Part model, mm, in its own coordinate system. Face numbers are marked on the shaded views. A direction names the side the tool comes from. Coordinates: 2 decimals unless noted, no trailing zeros. Order: outer loops, then holes, each group sorted by start corner. A loop starts at its lowest first (then second) coordinate and runs counter-clockwise, first axis right, second up. Notation, with made-up numbers: (14, 87.25) - (36, 87.25) arc R30 cw to (36, 110.25) - close; hole circle Ø5 at (7.5, -34). An arc over 180 degrees is marked (long way). Use a Markdown table: item, result. Add a question column.
1) Saw through at A-A on x = 44. List the corners of the cut face in (y, z), then the cut area to 3 significant figures.
2) Tool access for the marked faces 1, 2, 3, 4 and 5: list every direction of +Z, -Z, +X, -X, +Y, -Y with a clear straight run to the whole face (end or side of a thin tool).
3) Saw through at B-B on z = 10. List the corners of the cut face in (x, y).
4) Saw through at D-D on x = 30. List the corners of the cut face in (y, z), then the cut area to 3 significant figures.
5) Wall check: L1, parallel to X at y = 34.95, z = 15; L2, parallel to Z at x = 44, y = 34.15; L3, parallel to Y at x = 25.5, z = 16.5. Give the ranges that are in metal, low to high. Write a range as [from, to].
6) Saw through at C-C on y = 5. List the corners of the cut face in (x, z), then the cut area to 3 significant figures.
7) Drop flat-ended pins along their axis: P1, Ø5, axis at x = 38.5, z = 15.5, coming from the +Y side; P2, Ø1.5, axis at y = 38, z = 7, coming from the -X side; P3, Ø5.5, axis at x = -4.5, z = 8.5, coming from the +Y side; P4, Ø2, axis at x = -4, z = 11, coming from the -Y side. Give the stop position or say it passes through.
```python
from build123d import *

# Parameters (mm, degrees)
SKETCH1_W           = 40
SKETCH1_H           = 40.5
BOSS_EXTRUDE1_DEPTH = 20
SKETCH2_R           = 10
BOSS_EXTRUDE2_DEPTH = 6
SKETCH5_R           = 10
SKETCH5_R_2         = 5
CUT_EXTRUDE3_DEPTH  = 4
SKETCH6_W           = 20
SKETCH6_H           = 2
BOSS_EXTRUDE3_DEPTH = 7
SKETCH7_R           = 2
CUT_EXTRUDE5_DEPTH  = 2


with BuildPart() as part:
    # Sketch1 → Boss-Extrude1 (new body)
    with BuildSketch(Plane.XY):
        with Locations((20, 20.25)):
            Rectangle(SKETCH1_W, SKETCH1_H)
    extrude(amount=BOSS_EXTRUDE1_DEPTH)

    # Sketch2 → Boss-Extrude2 (add)
    with BuildSketch(Plane(origin=(0, 40.5, 0), x_dir=(1, 0, 0), z_dir=(0, 1, 0))):
        with Locations(Location((30, -10, 0), (0, 0, 270))):
            Circle(SKETCH2_R)
    extrude(amount=BOSS_EXTRUDE2_DEPTH)

    # Sketch5 → Cut-Extrude3 (cut)
    with BuildSketch(Plane(origin=(0, 40.5, 0), x_dir=(1, 0, 0), z_dir=(0, 1, 0))):
        with Locations(Location((30, -10, 0), (0, 0, 270))):
            Circle(SKETCH5_R)
        with Locations(Location((30, -10, 0), (0, 0, 270))):
            Circle(SKETCH5_R_2, mode=Mode.SUBTRACT)
    extrude(amount=CUT_EXTRUDE3_DEPTH, mode=Mode.SUBTRACT)

    # Sketch6 → Boss-Extrude3 (add)
    with BuildSketch(Plane.ZY):
        with Locations((10, 34.5)):
            Rectangle(SKETCH6_W, SKETCH6_H)
    boss_extrude3 = extrude(amount=BOSS_EXTRUDE3_DEPTH)

    # Sketch7 → Cut-Extrude5 (cut)
    with BuildSketch(Plane(origin=(0, 35.5, 0), x_dir=(1, 0, 0), z_dir=(0, 1, 0))):
        with Locations(Location((-4, -15, 0), (0, 0, 270))):
            Circle(SKETCH7_R)
        with Locations(Location((-4, -5, 0), (0, 0, 270))):
            Circle(SKETCH7_R)
    cut_extrude5 = extrude(amount=-CUT_EXTRUDE5_DEPTH, mode=Mode.SUBTRACT)

    # Mirror1: Boss-Extrude3, Cut-Extrude5 across plane
    add(boss_extrude3.mirror(Plane.ZY.offset(-20)))
    add(cut_extrude5.mirror(Plane.ZY.offset(-20)), mode=Mode.SUBTRACT)


solid = part.part
```
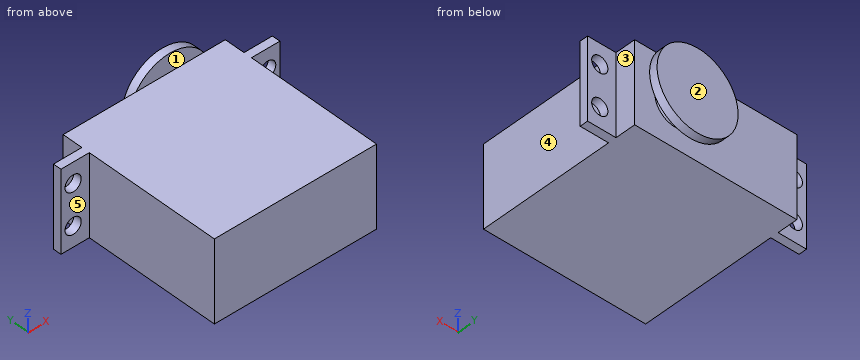
Results are:
| question | item | result |
|---|---|---|
| 1 | outline | (33.5, 0) - (35.5, 0) - (35.5, 3) - (33.5, 3) - close; (33.5, 7) - (35.5, 7) - (35.5, 13) - (33.5, 13) - close; (33.5, 17) - (35.5, 17) - (35.5, 20) - (33.5, 20) - close |
| 1 | area | 24.0 mm2 |
| 2 | face 1 | none |
| 2 | face 2 | +Z, -Z, +X, -X, +Y |
| 2 | face 3 | +Z, -Z, +X, +Y |
| 2 | face 4 | +Z, -Z, +X, -Y |
| 2 | face 5 | +Z, -Z, -X, -Y |
| 3 | outline | (-7, 33.5) - (0, 33.5) - (0, 0) - (40, 0) - (40, 33.5) - (47, 33.5) - (47, 35.5) - (40, 35.5) - (40, 40.5) - (35, 40.5) - (35, 44.5) - (40, 44.5) - (40, 46.5) - (20, 46.5) - (20, 44.5) - (25, 44.5) - (25, 40.5) - (0, 40.5) - (0, 35.5) - (-7, 35.5) - close |
| 4 | outline | (0, 0) - (40.5, 0) - (40.5, 5) - (44.5, 5) - (44.5, 0) - (46.5, 0) - (46.5, 20) - (44.5, 20) - (44.5, 15) - (40.5, 15) - (40.5, 20) - (0, 20) - close |
| 4 | area | 890 mm2 |
| 5 | L1 | [-7, -6], [-2, 42], [46, 47] |
| 5 | L2 | [0, 3], [7, 13], [17, 20] |
| 5 | L3 | [0, 40.5], [44.5, 46.5] |
| 6 | outline | (0, 0) - (40, 0) - (40, 20) - (0, 20) - close |
| 6 | area | 800 mm2 |
| 7 | P1 | y = 46.5 |
| 7 | P2 | x = 0 |
| 7 | P3 | y = 35.5 |
| 7 | P4 | y = 33.5 |
